Input: part model. Units: mm. Frame: model coordinates. Face numbers are marked on the shaded views. A direction names the side the tool comes from. Coordinates: 2 decimals unless noted, no trailing zeros. Loops run counter-clockwise (first coordinate to the right, second up) from the corner with the lowest first, then second, coordinate; pieces in that order, holes last. Notation, with made-up numbers: (-24, 23) -> (-5, 23) arc R15 cw to (-5, 30) -> close; hole circle Ø11 at (-27, -8). An arc over 180 degrees is marked (long way). Put each result on its own line as item: value. Start each with the question number.
1) Material intervals for L1, parallel to Y at x = 0, z = -102; L2, parallel to Y at x = 0, z = -93.5; L3, parallel to X at y = -67, z = -79, sorted ascending.
2) Set-up query: the marked faces 1, 2 and 3. Return all of +Z, -Z, +X, -X, +Y, -Y with unobstructed straight access to the full face (end or side cutting, diameter ignored); none if empty.
3) Cut plane C-C (z = -79.5). Return the cut outline in (x, y), plus the area to 3 significant figures.
4) Cut plane A-A (x = 0). Return the cut outline in (y, z), plus the area to 3 significant figures.
5) Pull-direction query (X, two-part tool) for the marked faces 4, 5 and 6; classes: pulls with the +X half, pulls with the -X half, needs draft (parallel to the pull), parting line crosses it, or undercut.
6) Contact query for flat-ended pins moving along their axis: P1, Ø6, axis at x = -16, z = -76.5, coming from the +Y side; P2, Ø20.5, axis at x = 3.5, y = -43.5, coming from the -Z side; P3, Ø3, axis at x = 17.5, z = -82, coming from the -Y side. Output: stop coordinate, or through.
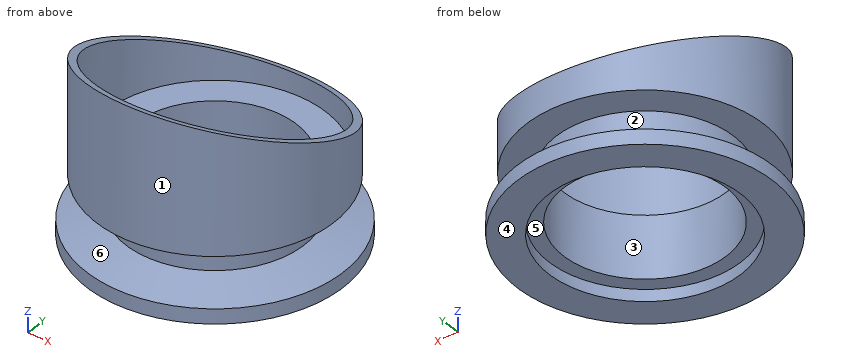
from build123d import *

# Parameters (mm, degrees)
CUT_EXTRUDE1_DEPTH      = 133.374626451
CUT_EXTRUDE1_DEPTH_BACK = 133.374626451


with BuildPart() as part:
    # Sketch4 → Revolve2 (revolve)
    with BuildSketch(Plane(origin=(0, 0, 0), x_dir=(0, 0, -1), z_dir=(1, 0, 0)), mode=Mode.PRIVATE) as revolve2_sk:
        Polygon((87.3252, -33.3375), (100.6602, -33.3375), (100.6602, -30.226), (103.2002, -30.226), (103.2002, -23.368), (100.0252, -23.368), (97.779249869, -31.75), (90.5002, -31.75), (90.5002, -25.4), (58.7502, -25.4), (58.7502, -27.051), (87.3252, -27.051), align=None)
    revolve(revolve2_sk.sketch.rotate(Axis((0, -50.8, -87.3252), (0, 0, -1)), 90), axis=Axis((0, -50.8, -87.3252), (0, 0, -1)))

    # Sketch10 → Cut-Extrude1 (cut, two sides: drawn at the far end of the back side and taken through both)
    with BuildSketch(Plane(origin=(0, 0, 0), x_dir=(0, 0, -1), z_dir=(1, 0, 0)).offset(-CUT_EXTRUDE1_DEPTH_BACK)):
        Polygon((57.499707015, -88.281372884), (88.550292985, -13.318627116), (35.383859736, -13.318627116), (35.383859736, -88.281372884), align=None)
    extrude(amount=CUT_EXTRUDE1_DEPTH + CUT_EXTRUDE1_DEPTH_BACK, mode=Mode.SUBTRACT)


solid = part.part
Results found:
1. L1: y = -78.23 to -71.37, -30.23 to -23.37
1. L2: y = -69.85 to -68.26, -33.34 to -31.75
1. L3: x = -19.56 to -17.37, 17.37 to 19.56
2. face 1: +Z
2. face 2: none
2. face 3: +Z, -Z
3. outline: (-20.02, -35.17) arc R25.4 ccw (long way) to (20.02, -35.17) -> (17.88, -35.17) arc R23.75 cw (long way) to (-17.88, -35.17) -> close
3. area: 183 mm2
4. outline: (-78.23, -103.2) -> (-71.37, -103.2) -> (-71.37, -100.66) -> (-68.26, -100.66) -> (-68.26, -87.33) -> (-74.55, -87.33) -> (-74.55, -63.19) -> (-76.2, -62.5) -> (-76.2, -90.5) -> (-69.85, -90.5) -> (-69.85, -97.78) -> (-78.23, -100.03) -> close; (-33.34, -100.66) -> (-30.23, -100.66) -> (-30.23, -103.2) -> (-23.37, -103.2) -> (-23.37, -100.03) -> (-31.75, -97.78) -> (-31.75, -90.5) -> (-25.4, -90.5) -> (-25.4, -83.55) -> (-27.05, -82.86) -> (-27.05, -87.33) -> (-33.34, -87.33) -> close
4. area: 194 mm2
5. face 4: needs draft
5. face 5: undercut
5. face 6: parting line crosses it
6. P1: stops at y = -65.05
6. P2: stops at z = -100.66
6. P3: stops at y = -70.53
